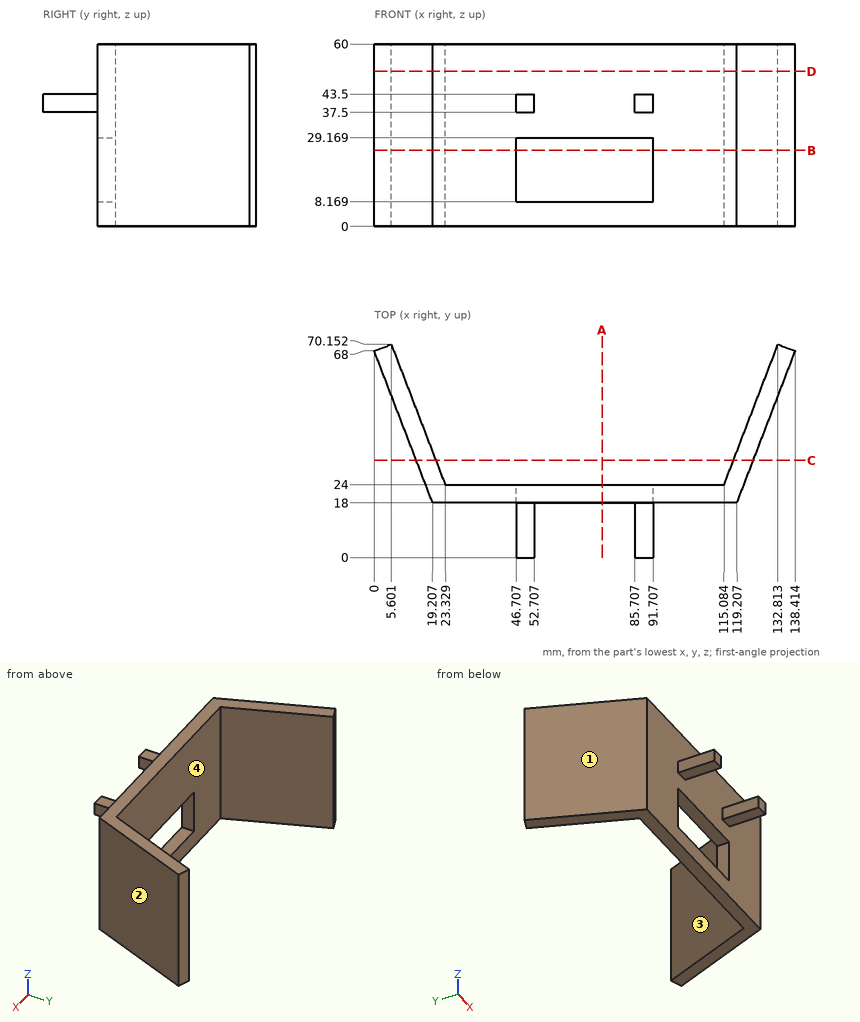
Design review of the part shown in the three views and the two pictorial views. Dimensions are in mm from the part's minimum x, y and z. Give positions to 0.01 mm unless a question says otherwise; leave off trailing zeros. Write each loop counter-clockwise with the first axis right and the second up, starting at its lowest first coordinate (ties: lowest second). Pieces come first, ordered by that corner, then holes. Notation, with made-up numbers: M 8,25.25 L 51,25.25 A31 cw 51,53.25 Z; hole C 34.25,38 d5. An arc over 180 degrees is marked long. Answer in a Markdown table with one row per item.
Item 1: Add section D-D on z = 51. Give the boundary of the cut face in (x, y) (1 decimal).
Check sheet entries:
| item | result |
|---|---|
| outline | M 0,68 L 19.2,18 L 119.2,18 L 138.4,68 L 132.8,70.2 L 115.1,24 L 23.3,24 L 5.6,70.2 Z |
Item 2: Add section A-A on x = 75. Give the boundary of the cut face in (y, z), plus the area to 3 significant figures.
Check sheet entries:
| item | result |
|---|---|
| outline | M 18,0 L 24,0 L 24,8.17 L 18,8.17 Z; M 18,29.17 L 24,29.17 L 24,60 L 18,60 Z |
| area | 234 mm2 |
Item 3: Draft analysis for pull direction X (two halves, no side actions). For the marked faces 1, 2, 3 and 4, state which applies: +X half, -X half, draft (parallel to the pull), parting line (faces both ways), or undercut.
Check sheet entries:
| item | result |
|---|---|
| face 1 | -X half |
| face 2 | +X half |
| face 3 | undercut |
| face 4 | undercut |
Item 4: For line 1 along X through (y, z) = (3, 38); line 2 along Y through (x, z) = (78.5, 56); line 3 along Z through (x, y) = (90.5, 20), list the stretches that pass through material, from the lowest coordinate up.
Check sheet entries:
| item | result |
|---|---|
| line 1 | 46.71 to 52.71, 85.71 to 91.71 |
| line 2 | 18 to 24 |
| line 3 | 0 to 8.17, 29.17 to 60 |
Item 5: For P1, Ø6.5, axis at y = 9.5, z = 40, coming from the -X side; P2, Ø3, axis at x = 49, y = 9.5, coming from the +Z side; P3, Ø3, axis at y = 5.5, z = 40, coming from the +X side, all flat-tipped, find the tip position at first contact; note any pin that passes through.
Check sheet entries:
| item | result |
|---|---|
| P1 | x = 46.71 |
| P2 | z = 43.5 |
| P3 | x = 91.71 |
Item 6: Add section B-B on z = 25. Give the boundary of the cut face in (x, y) (1 decimal).
Check sheet entries:
| item | result |
|---|---|
| outline | M 0,68 L 19.2,18 L 46.7,18 L 46.7,24 L 23.3,24 L 5.6,70.2 Z; M 91.7,18 L 119.2,18 L 138.4,68 L 132.8,70.2 L 115.1,24 L 91.7,24 Z |
Item 7: Add section C-C on y = 32. Give the boundary of the cut face in (x, z) (1 decimal).
Check sheet entries:
| item | result |
|---|---|
| outline | M 13.8,0 L 20.3,0 L 20.3,60 L 13.8,60 Z; M 118.2,0 L 124.6,0 L 124.6,60 L 118.2,60 Z |
